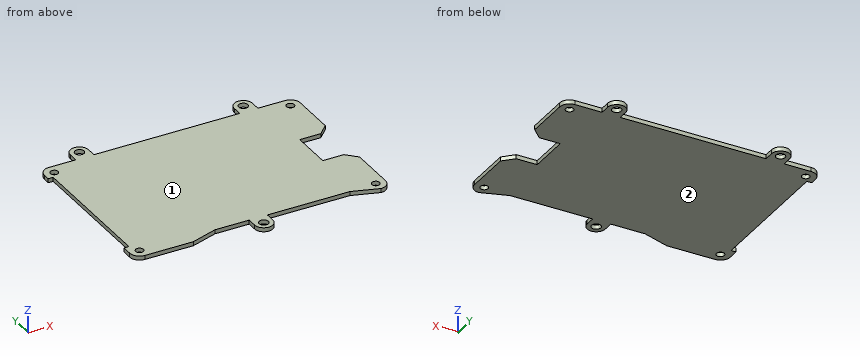
```python
from build123d import *

# Parameters (mm, degrees)
SKETCH1_R           = 1.355900406
BOSS_EXTRUDE1_DEPTH = 1.5875
SKETCH3_R           = 1.524
CUT_EXTRUDE1_DEPTH  = 430.891114182
SKETCH5_W           = 2.0955
SKETCH5_H           = 13.208
BOSS_EXTRUDE3_DEPTH = 1.5875
CUT_EXTRUDE2_DEPTH  = 430.891114182
SKETCH6_R           = 1.778
BOSS_EXTRUDE4_DEPTH = 1.5875


with BuildPart() as part:
    # Sketch1 → Boss-Extrude1 (new body)
    with BuildSketch(Plane.XY):
        with BuildLine():
            Line((-301.9473, 111.74645), (-305.87795, 115.6771))
            Line((-305.87795, 115.6771), (-316.1078, 115.6771))
            Line((-316.1078, 115.6771), (-316.1078, 128.8851))
            Line((-316.1078, 128.8851), (-305.87795, 128.8851))
            Line((-305.87795, 128.8851), (-301.9473, 132.81575))
            Line((-301.9473, 132.81575), (-301.9473, 150.9704))
            ThreePointArc((-301.9473, 150.9704), (-303.063223164, 153.664476836), (-305.7573, 154.7804))
            Line((-305.7573, 154.7804), (-397.247125, 154.7804))
            ThreePointArc((-397.247125, 154.7804), (-399.946077222, 153.659592612), (-401.0571, 150.956597849))
            Line((-401.0571, 150.956597849), (-401.0571, 148.341))
            Line((-401.0571, 148.341), (-399.1521, 148.341))
            Line((-399.1521, 148.341), (-399.1521, 95.6449))
            Line((-399.1521, 95.6449), (-401.0571, 95.6449))
            Line((-401.0571, 95.6449), (-401.0571, 91.659304166))
            ThreePointArc((-401.0571, 91.659304166), (-399.951018769, 88.947400452), (-397.2472, 87.8217))
            Line((-397.2472, 87.8217), (-378.5565, 87.8217))
            Line((-378.5565, 87.8217), (-368.3165, 91.1883))
            Line((-368.3165, 91.1883), (-315.9973, 91.1883))
            Line((-315.9973, 91.1883), (-305.7573, 87.8217))
            ThreePointArc((-305.7573, 87.8217), (-303.063223164, 88.937623164), (-301.9473, 91.6317))
            Line((-301.9473, 91.6317), (-301.9473, 111.74645))
        make_face()
        with Locations((-305.7573, 91.6317)):
            Circle(SKETCH1_R, mode=Mode.SUBTRACT)
        with Locations((-305.7573, 150.9704)):
            Circle(SKETCH1_R, mode=Mode.SUBTRACT)
        with Locations((-397.247125, 150.9704)):
            Circle(SKETCH1_R, mode=Mode.SUBTRACT)
        with Locations((-397.2472, 91.6317)):
            Circle(SKETCH1_R, mode=Mode.SUBTRACT)
    extrude(amount=BOSS_EXTRUDE1_DEPTH)

    # Sketch3 → Cut-Extrude1 (cut, through all)
    with BuildSketch(Plane.XY.offset(1.5875)):
        with Locations((-397.247125, 150.9704)):
            Circle(SKETCH3_R)
        with Locations((-305.7573, 150.9704)):
            Circle(SKETCH3_R)
        with Locations((-305.7573, 91.6317)):
            Circle(SKETCH3_R)
        with Locations((-397.2472, 91.6317)):
            Circle(SKETCH3_R)
    extrude(amount=-CUT_EXTRUDE1_DEPTH, mode=Mode.SUBTRACT)

    # Sketch5 → Boss-Extrude3 (add)
    with BuildSketch(Plane.XY.offset(1.5875)):
        with Locations((-315.06005, 122.2811)):
            Rectangle(SKETCH5_W, SKETCH5_H)
    extrude(amount=-BOSS_EXTRUDE3_DEPTH)

    # Sketch4 → Cut-Extrude2 (cut, through all)
    with BuildSketch(Plane.XY.offset(1.5875)):
        Polygon((-301.9473, 133.571034757), (-305.87795, 129.6471), (-314.0123, 129.6471), (-314.0123, 113.6451), (-305.87795, 113.6451), (-301.9473, 109.71445), align=None)
    extrude(amount=-CUT_EXTRUDE2_DEPTH, mode=Mode.SUBTRACT)

    # Sketch6 → Boss-Extrude4 (add)
    # profile 1 of 3: a face of its own
    with BuildSketch(Plane(origin=(0, 0, 0), x_dir=(-1, 0, 0), z_dir=(0, 0, -1))):
        with BuildLine():
            Line((386.7701125, 154.7804), (386.7701125, 158.5904))
            ThreePointArc((386.7701125, 158.5904), (383.2522125, 162.1083), (379.7343125, 158.5904))
            Line((379.7343125, 158.5904), (379.7343125, 154.7804))
            Line((379.7343125, 154.7804), (386.7701125, 154.7804))
        make_face()
        with Locations((383.2522125, 158.5904)):
            Circle(SKETCH6_R, mode=Mode.SUBTRACT)
    # profile 2 of 3: a face of its own
    with BuildSketch(Plane(origin=(0, 0, 0), x_dir=(-1, 0, 0), z_dir=(0, 0, -1))):
        with BuildLine():
            Line((347.9843125, 91.1883), (347.9843125, 87.3783))
            ThreePointArc((347.9843125, 87.3783), (351.5022125, 83.8604), (355.0201125, 87.3783))
            Line((355.0201125, 87.3783), (355.0201125, 91.1883))
            Line((355.0201125, 91.1883), (347.9843125, 91.1883))
        make_face()
        with Locations((351.5022125, 87.3783)):
            Circle(SKETCH6_R, mode=Mode.SUBTRACT)
    # profile 3 of 3: a face of its own
    with BuildSketch(Plane(origin=(0, 0, 0), x_dir=(-1, 0, 0), z_dir=(0, 0, -1))):
        with BuildLine():
            Line((316.2343125, 158.5904), (316.2343125, 154.7804))
            Line((316.2343125, 154.7804), (323.2701125, 154.7804))
            Line((323.2701125, 154.7804), (323.2701125, 158.5904))
            ThreePointArc((323.2701125, 158.5904), (319.7522125, 162.1083), (316.2343125, 158.5904))
        make_face()
        with Locations((319.7522125, 158.5904)):
            Circle(SKETCH6_R, mode=Mode.SUBTRACT)
    extrude(amount=-BOSS_EXTRUDE4_DEPTH)


solid = part.part
```
Work out the finished part from the listing and answer in its coordinate system (mm). Face numbers are marked on the shaded views. Round coordinates to 2 decimals unless told otherwise and drop trailing zeros. Loops run counter-clockwise (first coordinate to the right, second up) from the corner with the lowest first, then second, coordinate; pieces in that order, holes last.
(1) The part is cut by section C-C, the plane x = -357.5. Give the vertices of the cut face in (y, z).
Computed values:
outline: (91.19, 0) - (154.78, 0) - (154.78, 1.59) - (91.19, 1.59) - close
(2) The mould has two halves that part along Z. Classify the marked faces 1 and 2: pulls with the +Z half, pulls with the -Z half, needs draft (parallel to the pull), parting line crosses it, or undercut.
Computed values:
face 1: pulls with the +Z half
face 2: pulls with the -Z half
(3) The part is cut by section B-B, the plane y = 137. Give the vertices of the cut face in (x, z).
Computed values:
outline: (-399.15, 0) - (-301.95, 0) - (-301.95, 1.59) - (-399.15, 1.59) - close
(4) The part is cut by section A-A, the plane z = 1.2. Give the number of separate pieces and of enclosed holes in the cut face, and give its area (3 significant figures).
Computed values:
separate pieces: 1
enclosed holes: 7
area: 6,180 mm2
(5) Find the intervals of material crossed by L1, parallel to X at y = 128.5, z = 1; L2, parallel to X at y = 104, z = 0.3; L3, parallel to Y at x = -384, z = 0.5, in increasing order.
Computed values:
L1: x = -399.15 to -314.01
L2: x = -399.15 to -301.95
L3: y = 87.82 to 156.98, 160.2 to 162.03
(6) Each of these flat-tipped pins is pushed along its axis until it touches: P1, Ø2.5, axis at x = -305.76, y = 91.63, coming from the +Z side; P2, Ø0.8, axis at x = -400.5, z = 1, coming from the +Y side; P3, Ø0.5, axis at x = -309.5, z = 0.5, coming from the +Y side; P4, Ø0.5, axis at y = 156, z = 1, coming from the +X side. Where does it stop, or does it pass through?
Computed values:
P1: passes through
P2: stops at y = 153.5
P3: stops at y = 154.78
P4: stops at x = -316.23
